The drawing under review shows one solid part. Ordinate dimensions are in mm from its lowest x, y, z. A direction names the side the tool comes from. Give positions to 0.01 mm unless a question says otherwise; leave off trailing zeros. Write each loop counter-clockwise with the first axis right and the second up, starting at its lowest first coordinate (ties: lowest second). Pieces come first, ordered by that corner, then holes.
Q1. For line 1 (Y direction, x = 2.7, z = 4.45); line 2 (Z direction, x = 2.8, y = 3.5); line 3 (X direction, y = 6.5, z = 2.45), list the stretches that pass through material, from the lowest coordinate up.
Q2. We need section D-D (y = 7.25). Write out the cut boundary in (x, z), then the cut area to 3 significant figures.
Q3. Machinability: for the marked faces 4 and 5, which of the approach directions +Z, -Z, +X, -X, +Y, -Y give a long, thin tool a straight path to every point of the face, cutting with its end or side? Answer none if there is none.
Q4. We need section B-B (z = 2.75). Write out the cut boundary in (x, y), then the cut area to 3 significant figures.
Q5. We need section A-A (x = 2.75). Write out the cut boundary in (y, z).
Q6. We need section C-C (y = 3). Write out the cut boundary in (x, z).
Q7. Mouldability with a two-part tool opening along Y and no side actions: class the marked faces 1, 2 and 3 as released by +Y, released by -Y, zero draft, split by the parting line, or undercut.
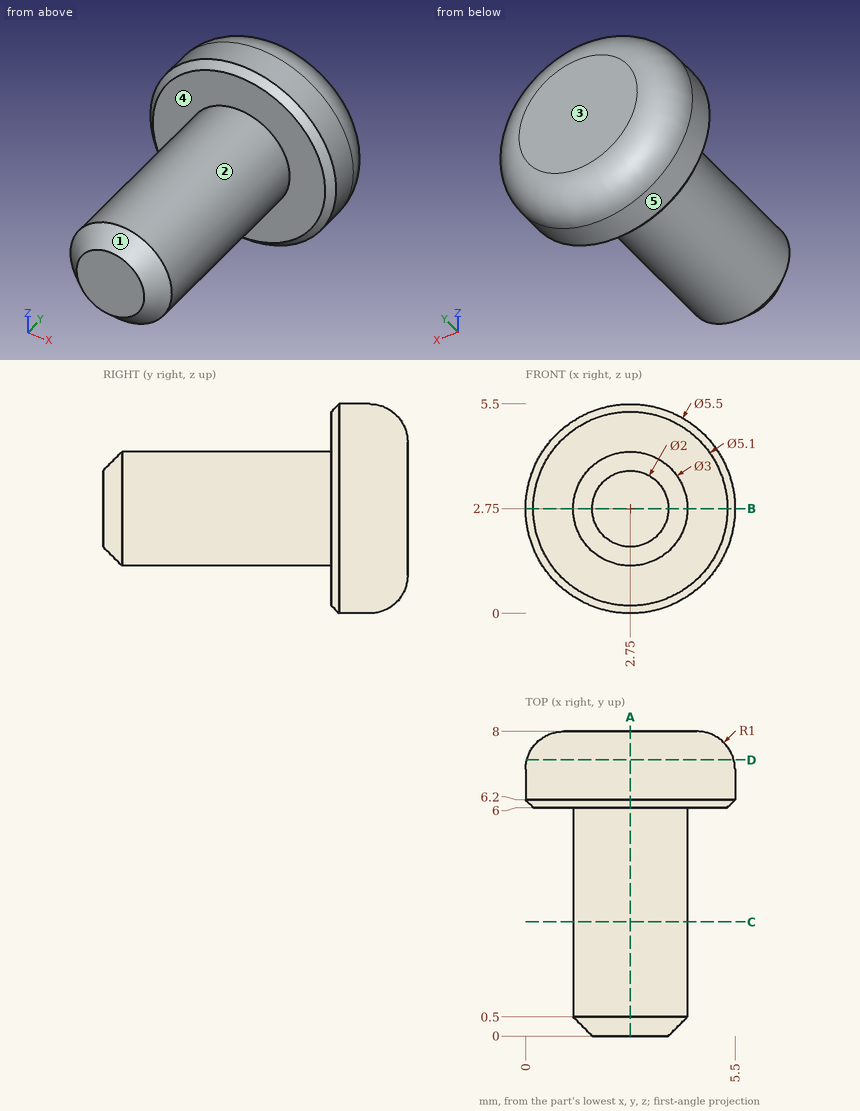
Computed:
1. line 1: y = 6 to 8
1. line 2: z = 1.25 to 4.25
1. line 3: x = 0.02 to 5.48
2. outline: circle Ø5.44 at (2.75, 2.75)
2. area: 23.2 mm2
3. face 4: -Y
3. face 5: +Y, -Y
4. outline: (0, 6.2) - (0.2, 6) - (1.25, 6) - (1.25, 0.5) - (1.75, 0) - (3.75, 0) - (4.25, 0.5) - (4.25, 6) - (5.3, 6) - (5.5, 6.2) - (5.5, 7) arc R1 ccw to (4.5, 8) - (1, 8) arc R1 ccw to (0, 7) - close
4. area: 28.3 mm2
5. outline: (0, 1.75) - (0.5, 1.25) - (6, 1.25) - (6, 0.2) - (6.2, 0) - (7, 0) arc R1 ccw to (8, 1) - (8, 4.5) arc R1 ccw to (7, 5.5) - (6.2, 5.5) - (6, 5.3) - (6, 4.25) - (0.5, 4.25) - (0, 3.75) - close
6. outline: circle Ø3 at (2.75, 2.75)
7. face 1: released by -Y
7. face 2: zero draft
7. face 3: released by +Y
